The listing builds one solid part. Answer for the finished solid, in the listing's coordinates (mm). Coordinates: 2 decimals unless noted, no trailing zeros. Order: outer loops, then holes, each group sorted by start corner. A loop starts at its lowest first (then second) coordinate and runs counter-clockwise, first axis right, second up.
from build123d import *

# Parameters (mm, degrees)
SKETCH2_W            = 82.5
SKETCH2_H            = 99
SKETCH2_R            = 0.8
SKETCH2_R_2          = 1.5
PCB_EXTRUDE_DEPTH    = 0.8
CORNER_FILLETS_R     = 1
SKETCH4_R            = 1.5
SOLAR_HOLES_DEPTH    = 2.6
SOLAR_HOLE_FILLETS_R = 0.5
M2_CLEARANCE_HOLES_D = 2.6
SKETCH10_W           = 1.75
SKETCH10_H           = 2.6
CUT_EXTRUDE2_DEPTH   = 2.6


with BuildPart() as part:
    # Sketch2 → pcb extrude (new body, symmetric)
    with BuildSketch(Plane.XY):
        Rectangle(SKETCH2_W, SKETCH2_H)
        with Locations((0, 46.95)):
            Circle(SKETCH2_R, mode=Mode.SUBTRACT)
        with Locations((-39.5, -30.25)):
            Circle(SKETCH2_R, mode=Mode.SUBTRACT)
        with Locations((-39.5, -0.25)):
            Circle(SKETCH2_R, mode=Mode.SUBTRACT)
        with Locations((-39.5, 29.75)):
            Circle(SKETCH2_R, mode=Mode.SUBTRACT)
        with Locations((39.5, -30.25)):
            Circle(SKETCH2_R, mode=Mode.SUBTRACT)
        with Locations((39.5, -0.25)):
            Circle(SKETCH2_R, mode=Mode.SUBTRACT)
        with Locations((39.5, 29.75)):
            Circle(SKETCH2_R, mode=Mode.SUBTRACT)
        with Locations((0, -46.95)):
            Circle(SKETCH2_R_2, mode=Mode.SUBTRACT)
        with Locations((-16.5, 20)):
            Circle(SKETCH2_R, mode=Mode.SUBTRACT)
        with Locations((16.5, 20)):
            Circle(SKETCH2_R, mode=Mode.SUBTRACT)
        with Locations((-16.5, -20)):
            Circle(SKETCH2_R, mode=Mode.SUBTRACT)
        with Locations((16.5, -20)):
            Circle(SKETCH2_R, mode=Mode.SUBTRACT)
    extrude(amount=PCB_EXTRUDE_DEPTH, both=True)

    # corner fillets
    corner_fillets_edges = [part.edges().sort_by_distance(p)[0] for p in [
        (41.25, 49.5, 0),
        (41.25, -49.5, 0),
        (-41.25, -49.5, 0),
        (-41.25, 49.5, 0),
    ]]
    fillet(corner_fillets_edges, radius=CORNER_FILLETS_R)

    # Sketch4 → solar holes (cut, through all)
    with BuildSketch(Plane.XY.offset(0.8)):
        with Locations((0, 46.95)):
            Circle(SKETCH4_R)
        with BuildLine():
            Line((6.2, 39.35), (-6.2, 39.35))
            Line((-6.2, 39.35), (-6.2, 46.65))
            Line((-6.2, 46.65), (-9.5, 46.65))
            ThreePointArc((-9.5, 46.65), (-10, 47.15), (-9.5, 47.65))
            Line((-9.5, 47.65), (-3, 47.65))
            Line((-3, 47.65), (-3, 44.15))
            Line((-3, 44.15), (3, 44.15))
            Line((3, 44.15), (3, 47.65))
            Line((3, 47.65), (9.5, 47.65))
            ThreePointArc((9.5, 47.65), (10, 47.15), (9.5, 46.65))
            Line((9.5, 46.65), (6.2, 46.65))
            Line((6.2, 46.65), (6.2, 39.35))
        make_face()
        with BuildLine():
            Line((6.2, -46.65), (9.5, -46.65))
            ThreePointArc((9.5, -46.65), (10, -47.15), (9.5, -47.65))
            Line((9.5, -47.65), (3, -47.65))
            Line((3, -47.65), (3, -44.15))
            Line((3, -44.15), (-3, -44.15))
            Line((-3, -44.15), (-3, -47.65))
            Line((-3, -47.65), (-9.5, -47.65))
            ThreePointArc((-9.5, -47.65), (-10, -47.15), (-9.5, -46.65))
            Line((-9.5, -46.65), (-6.2, -46.65))
            Line((-6.2, -46.65), (-6.2, -39.35))
            Line((-6.2, -39.35), (6.2, -39.35))
            Line((6.2, -39.35), (6.2, -46.65))
        make_face()
    extrude(amount=-SOLAR_HOLES_DEPTH, mode=Mode.SUBTRACT)

    # solar hole fillets
    solar_hole_fillets_edges = [part.edges().sort_by_distance(p)[0] for p in [
        (3, -47.65, 0),
        (3, -44.15, 0),
        (-3, -44.15, 0),
        (-3, -47.65, 0),
        (-6.2, -46.65, 0),
        (-6.2, -39.35, 0),
        (-6.2, 39.35, 0),
        (-6.2, 46.65, 0),
        (-3, 47.65, 0),
        (-3, 44.15, 0),
        (3, 44.15, 0),
        (3, 47.65, 0),
        (6.2, 46.65, 0),
        (6.2, 39.35, 0),
        (6.2, -39.35, 0),
        (6.2, -46.65, 0),
    ]]
    fillet(solar_hole_fillets_edges, radius=SOLAR_HOLE_FILLETS_R)

    # M2 Clearance Holes (through all)
    with Locations(Plane.XY.offset(0.8)):
        with Locations((-39.5, 29.75), (-39.5, -0.25), (-16.5, 20), (16.5, 20), (16.5, -20), (-16.5, -20), (39.5, 29.75), (39.5, -0.25), (39.5, -30.25), (-39.5, -30.25)):
            Hole(M2_CLEARANCE_HOLES_D / 2)

    # Sketch10 → Cut-Extrude2 (cut, through all)
    with BuildSketch(Plane.XY.offset(0.8)):
        with Locations((-40.375, 29.75)):
            Rectangle(SKETCH10_W, SKETCH10_H)
        with Locations((-40.375, -0.25)):
            Rectangle(SKETCH10_W, SKETCH10_H)
        with Locations((-40.375, -30.25)):
            Rectangle(SKETCH10_W, SKETCH10_H)
        with Locations((40.375, -30.25)):
            Rectangle(SKETCH10_W, SKETCH10_H)
        with Locations((40.375, -0.25)):
            Rectangle(SKETCH10_W, SKETCH10_H)
        with Locations((40.375, 29.75)):
            Rectangle(SKETCH10_W, SKETCH10_H)
    extrude(amount=-CUT_EXTRUDE2_DEPTH, mode=Mode.SUBTRACT)


solid = part.part
1) Consider L1, parallel to Y at x = 0, z = -0.2; L2, parallel to Y at x = -16.5, z = 0.2; L3, parallel to Y at x = 3.5, z = -0.35. Determine where each line is inside the solid, lowest interval first.
2) Section C-C (x = 16.5) is taken. Give the vertices of the cut face in (y, z), then the cut area to 3 significant figures.
3) Section A-A (y = 41) is taken. Give the vertices of the cut face in (x, z).
4) This flat-tipped pin is pushed along its axis until it touches: P1, Ø3.5, axis at x = -16.5, y = -20, coming from the +Z side. Where does it stop, or does it pass through?
5) Section D-D (z = -0.5) is taken. Give the number of separate pieces and of enclosed holes in the cut face, then the cut area to 3 significant figures.
6) Section B-B (y = -20) is taken. Give the vertices of the cut face in (x, z), then the cut area to 3 significant figures.
7) Determine the mould class of faces 1 (the face through (-0.195, 48.437, 0.011)), 2 (the face through (-1, 1, 0.8)), 3 (the face through (17.53, 19.21, -0.01)) for opening direction X: released by +X, released by -X, zero draft, split by the parting line, or undercut.
Filled sheet:
1. L1: y = -49.5 to -48.45, -45.45 to -44.15, -39.35 to 39.35, 44.15 to 45.45, 48.45 to 49.5
1. L2: y = -49.5 to -21.3, -18.7 to 18.7, 21.3 to 49.5
1. L3: y = -49.5 to -47.65, -39.35 to 39.35, 47.65 to 49.5
2. outline: (-49.5, -0.8) - (-21.3, -0.8) - (-21.3, 0.8) - (-49.5, 0.8) - close; (-18.7, -0.8) - (18.7, -0.8) - (18.7, 0.8) - (-18.7, 0.8) - close; (21.3, -0.8) - (49.5, -0.8) - (49.5, 0.8) - (21.3, 0.8) - close
2. area: 150 mm2
3. outline: (-41.25, -0.8) - (-6.2, -0.8) - (-6.2, 0.8) - (-41.25, 0.8) - close; (6.2, -0.8) - (41.25, -0.8) - (41.25, 0.8) - (6.2, 0.8) - close
4. P1: stops at z = 0.8
5. separate pieces: 1
5. enclosed holes: 8
5. area: 7,910 mm2
6. outline: (-41.25, -0.8) - (-17.8, -0.8) - (-17.8, 0.8) - (-41.25, 0.8) - close; (-15.2, -0.8) - (15.2, -0.8) - (15.2, 0.8) - (-15.2, 0.8) - close; (17.8, -0.8) - (41.25, -0.8) - (41.25, 0.8) - (17.8, 0.8) - close
6. area: 124 mm2
7. face 1: undercut
7. face 2: zero draft
7. face 3: undercut
